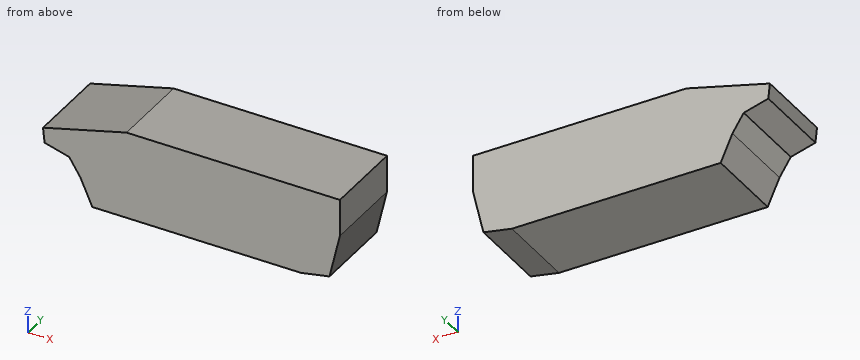
from build123d import *

# Parameters (mm, degrees)
F1_DEPTH = 70.000114


with BuildPart() as f1:
    # F0 (on Front) → F1 (new body)
    with BuildSketch(Plane.XZ):
        Polygon((140.789584, 39.61827), (-43.210302, 39.61827), (-115.23099, 20.556154), (-113.87212, 7.62737), (140.789584, 7.618334), align=None)
        Polygon((131.79156, -31.356391), (140.789584, 7.618334), (-113.87212, 7.62737), (-92.641751, 1.859206), (-82.917431, -13.287979), (-72.749014, -36.126616), (107.25088, -36.126616), align=None)
    extrude(amount=F1_DEPTH)


solid = f1.part
Can you work these out from the model? Positions are in its coordinate system, mm. Coordinates: 2 decimals unless noted, no trailing zeros. Write each loop counter-clockwise with the first axis right and the second up, starting at its lowest first coordinate (ties: lowest second). Pieces come first, ordered by that corner, then holes. Notation, with made-up numbers: (67, -18.5) - (77, -18.5) arc R36 cw to (77, 20.5) - close; hole circle Ø2 at (46.25, 88.25). An arc over 180 degrees is marked (long way). Return JSON: item names as keys, results as strings. Group by question number.
Item 1: If we section it at A-A (y = -32): Write out the boundary of the cut face in (x, z), then the cut area to 3 significant figures.
Item 2: I'm going to push flat-ended pins straight in: pin 1 Ø10 at (x, y) = (-73, -37.5) entering from +Z; pin 2 Ø1 at (y, z) = (-56.5, -1.5) entering from +X; pin 3 Ø5 at (y, z) = (-60.5, -28) entering from -X. Where does each tip first touch, or does it pass through?
Item 3: Please list where these lines run through material, in increasing order: probe 1 along X at (y, z) = (-65.5, 14.5); probe 2 along X at (y, z) = (-26.5, 12.5); probe 3 along Z at (x, y) = (-60.5, -58).
Item 4: If we section it at B-B (z = 30): Write out the boundary of the cut face in (x, y), then the cut area to 3 significant figures.
Item 5: If we section it at C-C (x = -54): Write out the boundary of the cut face in (y, z), then the cut area to 3 significant figures.
Return value:
{
 "1": {"outline": "(-115.23, 20.56) - (-113.87, 7.63) - (-92.64, 1.86) - (-82.92, -13.29) - (-72.75, -36.13) - (107.25, -36.13) - (131.79, -31.36) - (140.79, 7.62) - (140.79, 39.62) - (-43.21, 39.62) - close", "area": "17,100 mm^2"},
 "2": {"pin 1": "stops at z = 33.06", "pin 2": "stops at x = 138.8", "pin 3": "stops at x = -77.48"},
 "3": {"probe 1": "x = -114.59 to 140.79", "probe 2": "x = -114.38 to 140.79", "probe 3": "z = -36.13 to 35.04"},
 "4": {"outline": "(-79.55, -70) - (140.79, -70) - (140.79, 0) - (-79.55, 0) - close", "area": "15,400 mm^2"},
 "5": {"outline": "(-70, -36.13) - (0, -36.13) - (0, 36.76) - (-70, 36.76) - close", "area": "5,100 mm^2"}
}
